Build history of the part. All positions in model axes, mm. A direction names the side the tool comes from. Round coordinates to 2 decimals unless told otherwise and drop trailing zeros.
from build123d import *

# Parameters (mm, degrees)
BOSS_EXTRUDE1_DEPTH             = 12
BOSS_EXTRUDE1_DEPTH_BACK        = 44
BOSS_EXTRUDE2_REACH             = 56.729
BOSS_EXTRUDE2_DIRECTION_2_REACH = 56.729
CHAMFER1_SIZE                   = 0.75


# Read off the part's stored shape, not the designer's step: Sketch-Pattern1
with BuildPart() as part:
    # Sketch1 → Boss-Extrude1 (new, two sides: drawn at the far end of the back side and taken through both)
    with BuildSketch(Plane.XY.offset(-BOSS_EXTRUDE1_DEPTH_BACK)):
        Polygon((-13.75, 29.5), (13.75, 29.5), (13.75, 2.254), (11.21, 2.254), (11.21, 26.96), (-11.21, 26.96), (-11.21, 2.254), (-13.75, 2.254), align=None)
    extrude(amount=BOSS_EXTRUDE1_DEPTH + BOSS_EXTRUDE1_DEPTH_BACK)

    # Boss-Extrude2: up to this face of the body (flat: up to its plane)
    boss_extrude2_end = Plane(part.part.faces().sort_by_distance((13.75, 15.877, -16))[0])
    # Sketch2 → Boss-Extrude2 (add, up to the picked face)
    with BuildSketch(Plane(origin=(0, 0, 0), x_dir=(0, 0, -1), z_dir=(1, 0, 0)), mode=Mode.PRIVATE) as boss_extrude2_sk1:
        with BuildLine():
            Line((-3.872983346, 9), (-1, 20.127016654))
            ThreePointArc((-1, 20.127016654), (0, 28), (1, 20.127016654))
            Line((1, 20.127016654), (3.872983346, 9))
            ThreePointArc((3.872983346, 9), (0, 4), (-3.872983346, 9))
        make_face()
    boss_extrude2_tool1 = split(extrude(boss_extrude2_sk1.sketch, amount=BOSS_EXTRUDE2_REACH, mode=Mode.PRIVATE), bisect_by=boss_extrude2_end, keep=Keep.BOTH, mode=Mode.PRIVATE)
    # Sketch2 → Boss-Extrude2 (add, up to the picked face)
    with BuildSketch(Plane(origin=(0, 0, 0), x_dir=(0, 0, -1), z_dir=(1, 0, 0)), mode=Mode.PRIVATE) as boss_extrude2_sk2:
        with BuildLine():
            Line((-4.127016654, 17), (-6.698677596, 26.96))
            Line((-6.698677596, 26.96), (-9.301322404, 26.96))
            Line((-9.301322404, 26.96), (-11.872983346, 17))
            ThreePointArc((-11.872983346, 17), (-8, 12), (-4.127016654, 17))
        make_face()
    boss_extrude2_tool2 = split(extrude(boss_extrude2_sk2.sketch, amount=BOSS_EXTRUDE2_REACH, mode=Mode.PRIVATE), bisect_by=boss_extrude2_end, keep=Keep.BOTH, mode=Mode.PRIVATE)
    # Sketch2 → Boss-Extrude2 (add, up to the picked face)
    with BuildSketch(Plane(origin=(0, 0, 0), x_dir=(0, 0, -1), z_dir=(1, 0, 0)), mode=Mode.PRIVATE) as boss_extrude2_sk3:
        with BuildLine():
            Line((41.301322404, 26.96), (38.698677596, 26.96))
            Line((38.698677596, 26.96), (36.127016654, 17))
            ThreePointArc((36.127016654, 17), (40, 12), (43.872983346, 17))
            Line((43.872983346, 17), (41.301322404, 26.96))
        make_face()
    boss_extrude2_tool3 = split(extrude(boss_extrude2_sk3.sketch, amount=BOSS_EXTRUDE2_REACH, mode=Mode.PRIVATE), bisect_by=boss_extrude2_end, keep=Keep.BOTH, mode=Mode.PRIVATE)
    # Sketch2 → Boss-Extrude2 (add, up to the picked face)
    with BuildSketch(Plane(origin=(0, 0, 0), x_dir=(0, 0, -1), z_dir=(1, 0, 0)), mode=Mode.PRIVATE) as boss_extrude2_sk4:
        with BuildLine():
            Line((28.127016654, 9), (31, 20.127016654))
            ThreePointArc((31, 20.127016654), (32, 28), (33, 20.127016654))
            Line((33, 20.127016654), (35.872983346, 9))
            ThreePointArc((35.872983346, 9), (32, 4), (28.127016654, 9))
        make_face()
    boss_extrude2_tool4 = split(extrude(boss_extrude2_sk4.sketch, amount=BOSS_EXTRUDE2_REACH, mode=Mode.PRIVATE), bisect_by=boss_extrude2_end, keep=Keep.BOTH, mode=Mode.PRIVATE)
    add(boss_extrude2_tool1.solids().sort_by(Axis((0, 15.717101, 0), (1, 0, 0)))[0])
    add(boss_extrude2_tool2.solids().sort_by(Axis((0, 18.682958, 8), (1, 0, 0)))[0])
    add(boss_extrude2_tool3.solids().sort_by(Axis((0, 18.682958, -40), (1, 0, 0)))[0])
    add(boss_extrude2_tool4.solids().sort_by(Axis((0, 15.717101, -32), (1, 0, 0)))[0])

    # Boss-Extrude2 direction 2: up to this face of the body (flat: up to its plane)
    boss_extrude2_direction_2_end = Plane(part.part.faces().sort_by_distance((-13.75, 15.877, -16))[0])
    # Sketch2 → Boss-Extrude2 direction 2 (add, up to the picked face)
    with BuildSketch(Plane(origin=(0, 0, 0), x_dir=(0, 0, -1), z_dir=(1, 0, 0)), mode=Mode.PRIVATE) as boss_extrude2_direction_2_sk1:
        with BuildLine():
            Line((-3.872983346, 9), (-1, 20.127016654))
            ThreePointArc((-1, 20.127016654), (0, 28), (1, 20.127016654))
            Line((1, 20.127016654), (3.872983346, 9))
            ThreePointArc((3.872983346, 9), (0, 4), (-3.872983346, 9))
        make_face()
    boss_extrude2_direction_2_tool1 = split(extrude(boss_extrude2_direction_2_sk1.sketch, amount=-BOSS_EXTRUDE2_DIRECTION_2_REACH, mode=Mode.PRIVATE), bisect_by=boss_extrude2_direction_2_end, keep=Keep.BOTH, mode=Mode.PRIVATE)
    # Sketch2 → Boss-Extrude2 direction 2 (add, up to the picked face)
    with BuildSketch(Plane(origin=(0, 0, 0), x_dir=(0, 0, -1), z_dir=(1, 0, 0)), mode=Mode.PRIVATE) as boss_extrude2_direction_2_sk2:
        with BuildLine():
            Line((-4.127016654, 17), (-6.698677596, 26.96))
            Line((-6.698677596, 26.96), (-9.301322404, 26.96))
            Line((-9.301322404, 26.96), (-11.872983346, 17))
            ThreePointArc((-11.872983346, 17), (-8, 12), (-4.127016654, 17))
        make_face()
    boss_extrude2_direction_2_tool2 = split(extrude(boss_extrude2_direction_2_sk2.sketch, amount=-BOSS_EXTRUDE2_DIRECTION_2_REACH, mode=Mode.PRIVATE), bisect_by=boss_extrude2_direction_2_end, keep=Keep.BOTH, mode=Mode.PRIVATE)
    # Sketch2 → Boss-Extrude2 direction 2 (add, up to the picked face)
    with BuildSketch(Plane(origin=(0, 0, 0), x_dir=(0, 0, -1), z_dir=(1, 0, 0)), mode=Mode.PRIVATE) as boss_extrude2_direction_2_sk3:
        with BuildLine():
            Line((41.301322404, 26.96), (38.698677596, 26.96))
            Line((38.698677596, 26.96), (36.127016654, 17))
            ThreePointArc((36.127016654, 17), (40, 12), (43.872983346, 17))
            Line((43.872983346, 17), (41.301322404, 26.96))
        make_face()
    boss_extrude2_direction_2_tool3 = split(extrude(boss_extrude2_direction_2_sk3.sketch, amount=-BOSS_EXTRUDE2_DIRECTION_2_REACH, mode=Mode.PRIVATE), bisect_by=boss_extrude2_direction_2_end, keep=Keep.BOTH, mode=Mode.PRIVATE)
    # Sketch2 → Boss-Extrude2 direction 2 (add, up to the picked face)
    with BuildSketch(Plane(origin=(0, 0, 0), x_dir=(0, 0, -1), z_dir=(1, 0, 0)), mode=Mode.PRIVATE) as boss_extrude2_direction_2_sk4:
        with BuildLine():
            Line((28.127016654, 9), (31, 20.127016654))
            ThreePointArc((31, 20.127016654), (32, 28), (33, 20.127016654))
            Line((33, 20.127016654), (35.872983346, 9))
            ThreePointArc((35.872983346, 9), (32, 4), (28.127016654, 9))
        make_face()
    boss_extrude2_direction_2_tool4 = split(extrude(boss_extrude2_direction_2_sk4.sketch, amount=-BOSS_EXTRUDE2_DIRECTION_2_REACH, mode=Mode.PRIVATE), bisect_by=boss_extrude2_direction_2_end, keep=Keep.BOTH, mode=Mode.PRIVATE)
    add(boss_extrude2_direction_2_tool1.solids().sort_by(Axis((0, 15.717101, 0), (-1, 0, 0)))[0])
    add(boss_extrude2_direction_2_tool2.solids().sort_by(Axis((0, 18.682958, 8), (-1, 0, 0)))[0])
    add(boss_extrude2_direction_2_tool3.solids().sort_by(Axis((0, 18.682958, -40), (-1, 0, 0)))[0])
    add(boss_extrude2_direction_2_tool4.solids().sort_by(Axis((0, 15.717101, -32), (-1, 0, 0)))[0])


with BuildPart() as body_2:
    # Sketch5 → Revolve1 (revolve)
    with BuildSketch(Plane.XY.offset(8), mode=Mode.PRIVATE) as revolve1_sk:
        Polygon((6.13, 17.905), (6.13, 18.3495), (9.936012309, 18.3495), (13.75, 18.6162), (13.75, 16), (-13.75, 16), (-13.75, 18.6162), (-9.936012309, 18.3495), (-6.13, 18.3495), (-6.13, 17.905), align=None)
    revolve(revolve1_sk.sketch.rotate(Axis((0, 16, 8), (1, 0, 0)), 90), axis=Axis((0, 16, 8), (1, 0, 0)))


with BuildPart() as body_3:
    # Sketch-Pattern1 outline → Sketch-Pattern1 (revolve)
    with BuildSketch(Plane(origin=(0, 16, -40), x_dir=(0, 1, 0), z_dir=(0, 0, -1))):
        Polygon((0, 13.75), (0, -13.75), (2.6162, -13.75), (2.3495, -9.936012309), (2.3495, -6.13), (1.905, -6.13), (1.905, 6.13), (2.3495, 6.13), (2.3495, 9.936012309), (2.6162, 13.75), align=None)
    revolve(axis=Axis((0, 16, -40), (1, 0, 0)))


with BuildPart() as body_4:
    # Sketch-Pattern1 2 outline → Sketch-Pattern1 2 (revolve)
    with BuildSketch(Plane(origin=(0, 8, -32), x_dir=(0, 1, 0), z_dir=(0, 0, -1))):
        Polygon((0, 13.75), (0, -13.75), (2.6162, -13.75), (2.3495, -9.936012309), (2.3495, -6.13), (1.905, -6.13), (1.905, 6.13), (2.3495, 6.13), (2.3495, 9.936012309), (2.6162, 13.75), align=None)
    revolve(axis=Axis((0, 8, -32), (1, 0, 0)))


with BuildPart() as body_5:
    # Sketch-Pattern1 3 outline → Sketch-Pattern1 3 (revolve)
    with BuildSketch(Plane(origin=(0, 24, -32), x_dir=(0, 1, 0), z_dir=(0, 0, -1))):
        Polygon((0, 13.75), (0, -13.75), (2.6162, -13.75), (2.3495, -9.936012309), (2.3495, -6.13), (1.905, -6.13), (1.905, 6.13), (2.3495, 6.13), (2.3495, 9.936012309), (2.6162, 13.75), align=None)
    revolve(axis=Axis((0, 24, -32), (1, 0, 0)))


with BuildPart() as body_6:
    # Sketch-Pattern1 4 outline → Sketch-Pattern1 4 (revolve)
    with BuildSketch(Plane(origin=(0, 8, 0), x_dir=(0, 1, 0), z_dir=(0, 0, -1))):
        Polygon((0, 13.75), (0, -13.75), (2.6162, -13.75), (2.3495, -9.936012309), (2.3495, -6.13), (1.905, -6.13), (1.905, 6.13), (2.3495, 6.13), (2.3495, 9.936012309), (2.6162, 13.75), align=None)
    revolve(axis=Axis((0, 8, 0), (1, 0, 0)))


with BuildPart() as body_7:
    # Sketch-Pattern1 5 outline → Sketch-Pattern1 5 (revolve)
    with BuildSketch(Plane(origin=(0, 24, 0), x_dir=(0, 1, 0), z_dir=(0, 0, -1))):
        Polygon((0, 13.75), (0, -13.75), (2.6162, -13.75), (2.3495, -9.936012309), (2.3495, -6.13), (1.905, -6.13), (1.905, 6.13), (2.3495, 6.13), (2.3495, 9.936012309), (2.6162, 13.75), align=None)
    revolve(axis=Axis((0, 24, 0), (1, 0, 0)))


with BuildPart() as part_1:
    add(part.part)

    # Combine1: cut body 2, body 7, body 6, body 5, body 4, body 3
    add(body_2.part, mode=Mode.SUBTRACT)
    add(body_7.part, mode=Mode.SUBTRACT)
    add(body_6.part, mode=Mode.SUBTRACT)
    add(body_5.part, mode=Mode.SUBTRACT)
    add(body_4.part, mode=Mode.SUBTRACT)
    add(body_3.part, mode=Mode.SUBTRACT)

    # Chamfer1
    chamfer1_edges = [part_1.edges().sort_by_distance(p)[0] for p in [
        (-13.75, 2.254, -16),
        (13.75, 2.254, -16),
    ]]
    chamfer(chamfer1_edges, length=CHAMFER1_SIZE)


solid = part_1.part
1) Slice it at B-B (y = 8). Count the separate pieces of the cut face and the enclosed holes in it, plus the area to 3 significant figures.
Results:
separate pieces: 3
enclosed holes: 1
area: 402 mm2
2) Wall check: L1, parallel to Z at x = -1.5, y = 8 (3 decimals); L2, parallel to Y at x = 11.5, z = -33; L3, parallel to X at y = 26, z = -38. Give the ranges that are in metal, low to high.
Results:
L1: z = -36 to -33.905, -30.095 to -28, -4 to -1.905, 1.905 to 4
L2: y = 2.25 to 5.75, 10.25 to 21.75, 26.25 to 29.5
L3: x = -13.75 to -11.21, 11.21 to 13.75
3) Pin check, flat tips, straight feed: pin 1 Ø2 at (x, y) = (4, 22.5) entering from +Z; pin 2 Ø2 at (x, z) = (-1, -19) entering from -Y; pin 3 Ø1.4 at (y, z) = (7, -1) entering from -X. Stop position of each tip, or through.
Results:
pin 1: stops at z = 10.71
pin 2: stops at y = 26.96
pin 3: stops at x = -6.13
4) Which spindle directions (+Z, -Z, +X, -X, +Y, -Y) get a long thin tool onto all of the face, cutting with end or side? Do faces 3 (the cylindrical face through (8.06, 14.41, 6.27)), 4 (the cylindrical face through (0.157, 22.981, -28.132)), 5 (the flat face through (-11.21, 24, 11)). Say none if no direction does.
Results:
face 3: +X
face 4: none
face 5: +Z
5) Mould opens along Y. For faces 1 (the flat face through (0, 29.5, -16)), 2 (the flat face through (0, 26.96, 5)) say: released by +Y, released by -Y, zero draft, split by the parting line, or undercut.
Results:
face 1: released by +Y
face 2: undercut
